Geometry: final body of the model. Coordinates: model frame, mm. A direction names the side the tool comes from. Round coordinates to 2 decimals unless told otherwise and drop trailing zeros. Loops run counter-clockwise (first coordinate to the right, second up) from the corner with the lowest first, then second, coordinate; pieces in that order, holes last. Notation, with made-up numbers: M 79,6.5 L 129,6.5 A14 cw 129,13.5 Z; hole C -17,74 d5. An arc over 180 degrees is marked long. Return JSON: item names as keys, results as strings.
from build123d import *

# Parameters (mm, degrees)
BOSS_EXTRUDE1_DEPTH = 19
SKETCH2_W           = 33
SKETCH2_H           = 13
CUT_EXTRUDE1_DEPTH  = 3
CUT_EXTRUDE2_REACH  = 60.752
SKETCH3_W           = 23
SKETCH3_H           = 13


with BuildPart() as part:
    # Sketch1 → Boss-Extrude1 (new body)
    with BuildSketch(Plane.XY):
        Polygon((-29.283593539, 0), (29.283593539, 0), (43.14, -24), (49.14, -24), (32.396842194, 5), (-32.396842194, 5), (-49.14, -24), (-43.14, -24), align=None)
    extrude(amount=BOSS_EXTRUDE1_DEPTH)

    # Sketch2 → Cut-Extrude1 (cut)
    with BuildSketch(Plane(origin=(0, 5, 0), x_dir=(1, 0, 0), z_dir=(0, 1, 0))):
        with Locations((-5.8, -9.5)):
            Rectangle(SKETCH2_W, SKETCH2_H)
    extrude(amount=-CUT_EXTRUDE1_DEPTH, mode=Mode.SUBTRACT)

    # Sketch3 → Cut-Extrude2 (cut, up to next)
    with BuildSketch(Plane(origin=(0, 2, 0), x_dir=(1, 0, 0), z_dir=(0, 1, 0)), mode=Mode.PRIVATE) as cut_extrude2_sk1:
        with Locations((-5.8, -9.5)):
            Rectangle(SKETCH3_W, SKETCH3_H)
    cut_extrude2_tool1 = extrude(cut_extrude2_sk1.sketch, amount=-CUT_EXTRUDE2_REACH, mode=Mode.PRIVATE) & part.part
    add(cut_extrude2_tool1.solids().sort_by_distance((-5.8, 2, 9.5))[0], mode=Mode.SUBTRACT)


solid = part.part
Q1. Material intervals for L1, parallel to X at y = -10.25, z = 5; L2, parallel to Y at x = -27, z = 2; L3, parallel to X at y = -15.25, z = 5.25, sorted ascending.
Determined:
{"L1": "x = -41.2 to -35.2, 35.2 to 41.2", "L2": "y = 0 to 5", "L3": "x = -44.09 to -38.09, 38.09 to 44.09"}
Q2. Section query D-D (z = 17.25). Output: boundary loops of the cut face in (x, y), plus the area to 3 significant figures.
Determined:
{"outline": "M -49.14,-24 L -43.14,-24 L -29.28,0 L 29.28,0 L 43.14,-24 L 49.14,-24 L 32.4,5 L -32.4,5 Z", "area": "626 mm^2"}
Q3. Section query A-A (x = 2). Output: boundary loops of the cut face in (y, z).
Determined:
{"outline": "M 0,0 L 5,0 L 5,3 L 0,3 Z; M 0,16 L 5,16 L 5,19 L 0,19 Z"}
Q4. Reachability of faces 1 (the flat face through (-20, 2, 9)), 2 (the flat face through (5.7, 1, 10)), 3 (the flat face through (36.115, -11.832, 9.367)) from +Z, -Z, +X, -X, +Y, -Y: full face, straight path, thin tool, end or side. Return the list, or none.
Determined:
{"face 1": "+Y", "face 2": "+Y, -Y", "face 3": "+Z, -Z, -Y"}
Q5. Pin query (flat end, axial travel): pin 1 (1.5 mm diameter, centred on x = 9, z = 7, fed in from +Y); pin 2 (1 mm diameter, centred on y = 1, z = 6.5, fed in from -X); pin 3 (2.5 mm diameter, centred on y = 4, z = 10, fed in from -X). Return the tip coordinate at first contact, or that it passes through.
Determined:
{"pin 1": "stops at y = 2", "pin 2": "stops at x = -34.99", "pin 3": "stops at x = -33.7"}
Q6. Section query C-C (y = 1). Output: boundary loops of the cut face in (x, z), plus the area to 3 significant figures.
Determined:
{"outline": "M -34.71,0 L 34.71,0 L 34.71,19 L -34.71,19 Z; hole M -17.3,3 L 5.7,3 L 5.7,16 L -17.3,16 Z", "area": "1,020 mm^2"}
Q7. Section query B-B (z = 6.25). Output: boundary loops of the cut face in (x, y), plus the area to 3 significant figures.
Determined:
{"outline": "M -49.14,-24 L -43.14,-24 L -29.28,0 L -17.3,0 L -17.3,2 L -22.3,2 L -22.3,5 L -32.4,5 Z; M 5.7,0 L 29.28,0 L 43.14,-24 L 49.14,-24 L 32.4,5 L 10.7,5 L 10.7,2 L 5.7,2 Z", "area": "481 mm^2"}
Q8. Pull-direction query (Z, two-part tool) for faces 4 (the flat face through (-0.2, 0.2, 19)), 5 (the flat face through (-22.3, 4, 10)), 6 (the flat face through (-40.651, -9.297, 9.367)); classes: pulls with the +Z half, pulls with the -Z half, needs draft (parallel to the pull), parting line crosses it, or undercut.
Determined:
{"face 4": "pulls with the +Z half", "face 5": "undercut", "face 6": "needs draft"}
